The model under review builds one solid part; all positions refer to its coordinate system, in mm. Face numbers are marked on the shaded views. A direction names the side the tool comes from. Give positions to 0.01 mm unless a question says otherwise; leave off trailing zeros. Order: outer loops, then holes, each group sorted by start corner. A loop starts at its lowest first (then second) coordinate and runs counter-clockwise, first axis right, second up. Notation, with made-up numbers: (-7, 22) - (9, 22) arc R33 cw to (9, 59) - close; hole circle Ø4 at (64.5, 46.5). An arc over 180 degrees is marked (long way). Use CSV: the item, a comma, the result in double quotes.
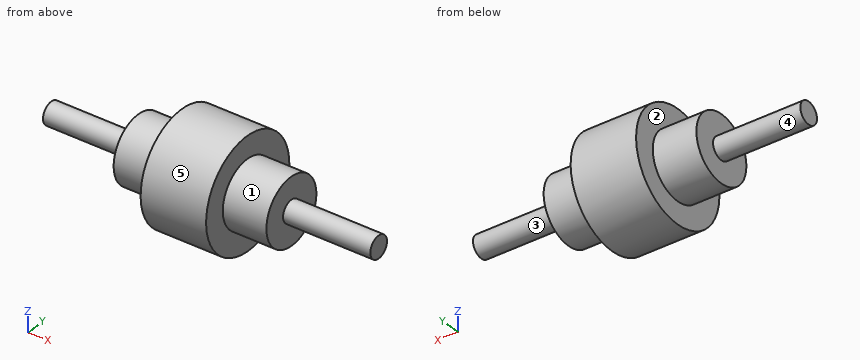
```python
from build123d import *


with BuildPart() as part:
    # Sketch2 → Revolve1 (revolve)
    with BuildSketch(Plane(origin=(0, 0, 0), x_dir=(1, 0, 0), z_dir=(0, 1, 0)), mode=Mode.PRIVATE) as revolve1_sk:
        Polygon((45.011364727, -30), (45.011364727, -50), (105.011364727, -50), (105.011364727, -30), (145.011364727, -30), (145.011364727, -10), (225.011364727, -10), (225.011364727, 0), (-74.988635273, 0), (-74.988635273, -10), (5.011364727, -10), (5.011364727, -30), align=None)
    revolve(revolve1_sk.sketch.rotate(Axis((0, 0, 0), (-1, 0, 0)), 180), axis=Axis((0, 0, 0), (-1, 0, 0)))  # turned: the seam where the file's is


solid = part.part
```
Item 1: Take a section at D-D, the plane y = -24.5. Give the boundary of the cut face in (x, z), and give its area (3 significant figures).
Results list:
outline,"(5.01, -17.31) - (45.01, -17.31) - (45.01, -43.59) - (105.01, -43.59) - (105.01, -17.31) - (145.01, -17.31) - (145.01, 17.31) - (105.01, 17.31) - (105.01, 43.59) - (45.01, 43.59) - (45.01, 17.31) - (5.01, 17.31) - close"
area,"8,000 mm2"
Item 2: Take a section at C-C, the plane x = 134. Give the boundary of the cut face in (y, z), and give its area (3 significant figures).
Results list:
outline,"circle Ø60 at (0, 0)"
area,"2,830 mm2"
Item 3: Tool access review of the marked faces 3, 4 and 5: name each direction out of +Z, -Z, +X, -X, +Y, -Y from which nothing blocks a thin tool from reaching the whole face with its end or side.
Results list:
face 3,"+X"
face 4,"-X"
face 5,"+X, -X"
Item 4: Clearance check with flat-ended pins moving along their axes: pin 1 (6 mm diameter, centred on x = 20.5, y = -1, fed in from +Z); pin 2 (1 mm diameter, centred on y = -21.5, z = -28.5, fed in from +X); pin 3 (1.5 mm diameter, centred on x = 167.5, y = -6.5, fed in from +Z). State where each tip first meets the part, or that it passes through.
Results list:
pin 1,"stops at z = 30"
pin 2,"stops at x = 105.01"
pin 3,"stops at z = 8.18"
Item 5: Take a section at A-A, the plane z = 0. Give the boundary of the cut face in (x, y), and give its area (3 significant figures).
Results list:
outline,"(-74.99, -10) - (5.01, -10) - (5.01, -30) - (45.01, -30) - (45.01, -50) - (105.01, -50) - (105.01, -30) - (145.01, -30) - (145.01, -10) - (225.01, -10) - (225.01, 10) - (145.01, 10) - (145.01, 30) - (105.01, 30) - (105.01, 50) - (45.01, 50) - (45.01, 30) - (5.01, 30) - (5.01, 10) - (-74.99, 10) - close"
area,"14,000 mm2"
Item 6: Mouldability with a two-part tool opening along Y and no side actions: class the marked faces 1 and 2 as pulls with the +Y half, pulls with the -Y half, needs draft (parallel to the pull), parting line crosses it, or undercut.
Results list:
face 1,"parting line crosses it"
face 2,"needs draft"
Item 7: Wall thickness on L1, parallel to X at y = 20, z = -23.5; L2, parallel to X at y = 14, z = -0.5; L3, parallel to Y at x = 53, z = 8: over which ranges is each line inside the solid? List them lowest first.
Results list:
L1,"x = 45.01 to 105.01"
L2,"x = 5.01 to 145.01"
L3,"y = -49.36 to 49.36"
Item 8: Take a section at B-B, the plane y = -5.5. Give the boundary of the cut face in (x, z).
Results list:
outline,"(-74.99, -8.35) - (5.01, -8.35) - (5.01, -29.49) - (45.01, -29.49) - (45.01, -49.7) - (105.01, -49.7) - (105.01, -29.49) - (145.01, -29.49) - (145.01, -8.35) - (225.01, -8.35) - (225.01, 8.35) - (145.01, 8.35) - (145.01, 29.49) - (105.01, 29.49) - (105.01, 49.7) - (45.01, 49.7) - (45.01, 29.49) - (5.01, 29.49) - (5.01, 8.35) - (-74.99, 8.35) - close"
